Autodesk Inventor part; units mm, degrees
ref_plane "YZ Plane" through (0, 0, 0) normal (1, 0, 0) x (0, 1, 0)
ref_plane "XZ Plane" through (0, 0, 0) normal (0, 1, 0) x (-1, 0, 0)
ref_plane "XY Plane" through (0, 0, 0) normal (0, 0, 1) x (1, 0, 0)
sketch "Sketch1" plane through (0, 0, 0) normal (0, 1, 0) x (-1, 0, 0)
  line L0 (0, 0) -> (0, -31.748)
  line L1 (0, -31.748) -> (7.62, -31.748)
  line L2 (7.62, -31.748) -> (7.62, -26.16)
  line L3 (7.62, -26.16) -> (4.953, -26.16)
  line L4 (4.953, -26.16) -> (4.953, -23.493)
  line L5 (4.953, -23.493) -> (7.62, -23.493)
  line L6 (7.62, -23.493) -> (7.62, -17.016)
  line L7 (7.62, -17.016) -> (2.54, -17.016)
  line L8 (2.54, -17.016) -> (2.54, 0)
  line L9 (0, 0) -> (2.54, 0)
  dimension "d0" = 31.748
  dimension "d1" = 7.62
  dimension "d2" = 5.588
  dimension "d3" = 2.667
  dimension "d4" = 2.667
  dimension "d5" = 6.477
  dimension "d6" = 5.08
  dimension "d7" = 2.54
revolve "Revolution1" add sketch "Sketch1" angle 360 about axis through (0, 0, 0) along (-1, 0, 0)
sketch "Sketch2" plane through (-7.62, 0, 0) normal (-1, 0, 0) x (0, 0, 1)
  circle A0 centre (28.954, 0) radius 1.5
  circle A1 centre (0, 0) radius 31.748
  line L0 (31.748, 0) -> (26.16, 0)
  circle A2 centre (0, 0) radius 26.16
  circle A3 centre (0, 28.954) radius 1.5
  circle A4 centre (-28.954, 0) radius 1.5
  circle A5 centre (0, -28.954) radius 1.5
  dimension "d9" = 3
  dimension "d12" = 360
extrude "Extrusion1" cut sketch "Sketch2" against normal blind 12.7 contours L0 A0 | A0 L0 | A3 | A4 | A5
sketch "Sketch3" plane through (0, 0, 0) normal (1, 0, 0) x (0, 0, -1)
  circle A0 centre (0, 0) radius 23.493
  circle A1 centre (0, 0) radius 20.2545
  circle A2 centre (20.2545, 0) radius 1.5
  circle A3 centre (0, 20.2545) radius 1.5
  circle A4 centre (-20.2545, 0) radius 1.5
  circle A5 centre (0, -20.2545) radius 1.5
  dimension "d17" = 3.2385
  dimension "d18" = 3
  dimension "d21" = 360
sketch "Sketch4" plane through (-7.62, 0, 0) normal (-1, 0, 0) x (0, 0, 1)
  circle A0 centre (0, 0) radius 17.016
  circle A1 centre (0, 0) radius 23.493
  dimension "d16" = 6.477
extrude "Extrusion2" cut sketch "Sketch3" against normal blind 5.08 contours A1 A2 | A1 A2 | A3 A1 | A1 A3 | A5 A1 | A1 A5 | A4 A1 | A1 A4
sketch "Sketch5" plane through (-2.54, 0, 0) normal (-1, 0, 0) x (0, 0, 1)
  circle A0 centre (0, 0) radius 17.016
  line L0 (-17.016, 0) -> (17.016, 0)
  line L1 (-14.478, -9.9949) -> (14.478, -9.9949)
  line L2 (-14.478, 9.9949) -> (14.478, 9.9949)
  line L3 (14.478, 9.9949) -> (14.478, -9.9949)
  line L4 (-14.478, 9.9949) -> (-14.478, -9.9949)
  arc A1 (16.8267, -2.5309) -> (16.8267, 2.5309) centre (0, 0) ccw
  point P0 (0, 9.9949)
  point P1 (14.478, 0)
  dimension "d25" = 28.956
  dimension "d26" = 19.9898
sketch "Sketch8" plane through (-7.62, 0, 0) normal (-1, 0, 0) x (0, 0, 1)
  arc A0 (-17.016, 0) -> (-17.016, 0) centre (17.016, 0) ccw
  arc A1 (-16.8238, -2.55) -> (-16.829, 2.5158) centre (-17.016, -0.0173) ccw
  circle A2 centre (-14.476, -0.0173) radius 2.54
  circle A3 centre (14.476, 0) radius 2.54
  point P0 (0, 0)
extrude "Extrusion4" cut sketch "Sketch8" against normal blind 25.4 contours A2 A1 | A2 A1 | A3
properties part number "LED holder 2"
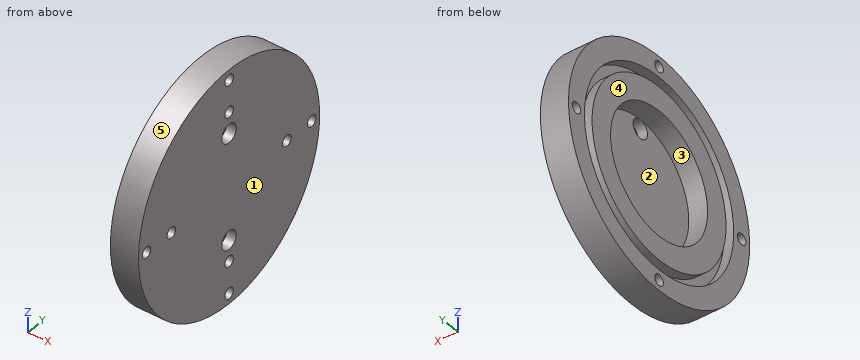
Read the model definition and answer for the solid it produces. Units are mm, in the model's axes. Face numbers are marked on the shaded views. A direction names the side the tool comes from. Give positions to 0.01 mm unless a question says otherwise; leave off trailing zeros. Write each loop counter-clockwise with the first axis right and the second up, starting at its lowest first coordinate (ties: lowest second). Pieces come first, ordered by that corner, then holes. Notation, with made-up numbers: M -15.5,-16 L 10.5,-16 A13 ccw 10.5,-10 Z; hole C 60,-0.75 d4. An arc over 180 degrees is marked long. Put each result on its own line as item: value. Start each with the question number.
1. The part is cut by section C-C, the plane z = -14. Give the vertices of the cut face in (x, y), and give its area (3 significant figures).
2. The part is cut by section A-A, the plane z = 0. Give the number of separate pieces and of enclosed holes in the cut face, and give its area (3 significant figures).
3. Which of the six approach directions +Z, -Z, +X, -X, +Y, -Y give full straight-line access (tool end or side, diameter ignored) to the marked faces 1 and 2?
4. The part is cut by section B-B, the plane x = -6.5. Give the vertices of the cut face in (y, z).
5. Consider line 1 along Y through (x, z) = (-4, 0); line 2 along Y through (x, z) = (-5.8, 0); line 3 along Y through (x, z) = (-6.5, 15.5). Determine where each line is inside the solid, lowest interval first.
6. Each of these flat-tipped pins is pushed along its axis until it touches: pin 1 Ø1.5 at (x, y) = (-5.5, -23.5) entering from -Z; pin 2 Ø1 at (x, y) = (-5.5, 7.5) entering from +Z; pin 3 Ø0.9 at (y, z) = (-20.5, 0) entering from +X. Where does it stop, or does it pass through?
7. The part is cut by section D-D, the plane y = -24.5. Give the vertices of the cut face in (x, z), and give its area (3 significant figures).
8. For a pull along Z with two mould halves and no side action, classify the marked faces 3, 4 and 5 as released by +Z, released by -Z, zero draft, split by the parting line, or undercut.
Final values:
1. outline: M -7.62,-28.49 L 0,-28.49 L 0,-2.51 L -2.54,-2.51 L -2.54,-9.67 L -7.62,-9.67 L -7.62,-18.87 L -4.95,-18.87 L -4.95,-22.1 L -7.62,-22.1 Z; M -7.62,9.67 L -2.54,9.67 L -2.54,2.48 L 0,2.48 L 0,28.49 L -7.62,28.49 L -7.62,22.1 L -4.95,22.1 L -4.95,18.87 L -7.62,18.87 Z
1. area: 306 mm²
2. separate pieces: 3
2. enclosed holes: 0
2. area: 221 mm²
3. face 1: +Z, -Z, +X, +Y, -Y
3. face 2: -X
4. outline: C 0,0 d63.5; C 0,0 d46.99; hole C -28.95,0 d3; hole C 0,0 d52.32; hole C 0,0 d34.03; hole C 0,-28.95 d3; hole C 0,28.95 d3; hole C 28.95,0 d3
5. line 1: y = -31.75 to -30.45, -27.45 to -21.75, -18.75 to -17.02, 17.02 to 18.75, 21.75 to 27.45, 30.45 to 31.75
5. line 2: y = -31.75 to -30.45, -27.45 to -26.16, -23.49 to -17.02, 17.02 to 23.49, 26.16 to 27.45, 30.45 to 31.75
5. line 3: y = -27.71 to -21.07, -17.65 to -7.02, 7.02 to 17.65, 21.07 to 27.71
6. pin 1: stops at z = -22.14
6. pin 2: stops at z = 30.97
6. pin 3: stops at x = -5.08
7. outline: M -7.62,-20.19 L 0,-20.19 L 0,20.19 L -7.62,20.19 L -7.62,9.17 L -4.95,9.17 L -4.95,-9.17 L -7.62,-9.17 Z
7. area: 259 mm²
8. face 3: undercut
8. face 4: zero draft
8. face 5: split by the parting line
